from build123d import *

# Parameters (mm, degrees)
F2_R     = 2
F3_R     = 2
F4_R     = 4.6529317806
F4_R_2   = 2.3810630886
F5_DEPTH = 2.1


# Not quite as in the source:
# - a feature names something its author has since deleted; it is built from what else it names


with BuildPart() as f1:
    # F0 (on Top) → F1 (revolve)
    with BuildSketch(Plane.XY):
        with BuildLine():
            Line((12, 0), (5, 0))
            Line((5, 0), (5, 23.4674374053))
            ThreePointArc((5, 23.4674374053), (5.4354487572, 25.0240609703), (6.6153846154, 26.1287980041))
            ThreePointArc((6.6153846154, 26.1287980041), (10.5485041427, 29.8112547834), (12, 35))
            Line((12, 35), (12, 35.8777977526))
            ThreePointArc((12, 35.8777977526), (11.6461494723, 39.1166718836), (10.6012925819, 42.2027357051))
            Line((10.6012925819, 42.2027357051), (2.7202585164, 59.1502932902))
            ThreePointArc((2.7202585164, 59.1502932902), (1.6132323497, 60.414629994), (0, 60.8853056997))
            Line((0, 60.8853056997), (0, 25))
            Line((0, 25), (0, 17.2050446272))
            Line((0, 17.2050446272), (0, -4))
            Line((0, -4), (9, -4))
            Line((9, -4), (12, -4))
            Line((12, -4), (12, 0))
        make_face()
    revolve(axis=Axis((0, 21.1025223136, 0), (0, -1, 0)))

    # F2
    f2_edges = [f1.edges().sort_by_distance(p)[0] for p in [
        (-12, 0, 0),
    ]]
    fillet(f2_edges, radius=F2_R)

    # F3
    f3_edges = [f1.edges().sort_by_distance(p)[0] for p in [
        (-5, 0, 0),
    ]]
    fillet(f3_edges, radius=F3_R)

    # F4 (on Top) → F5 (cut, symmetric)
    with BuildSketch(Plane.XY):
        with Locations((0, -4.1621848941)):
            Circle(F4_R)
        with Locations((0, -4.1621848941)):
            Circle(F4_R_2, mode=Mode.SUBTRACT)
    extrude(amount=F5_DEPTH, both=True, mode=Mode.SUBTRACT)


solid = f1.part
Could you check a few things on this model? Use its own coordinates, in mm. A direction names the side the tool comes from. Round coordinates to 2 decimals unless told otherwise and drop trailing zeros. Order: outer loops, then holes, each group sorted by start corner. A loop starts at its lowest first (then second) coordinate and runs counter-clockwise, first axis right, second up.
Q1. Imagine slicing it at A-A, the plane y = 21. List the corners of the cut face in (x, z) for me.
Geometry says:
outline: circle Ø10 at (0, 0)
Q2. Please list where these lines run through material, in increasing order: probe 1 along Y at (x, z) = (-5.5, -3.75); probe 2 along Y at (x, z) = (-2, 8.75); probe 3 along X at (y, z) = (53, -2.5).
Geometry says:
probe 1: y = -4 to 0.03, 26.15 to 50.69
probe 2: y = -4 to 0, 27.83 to 45.7
probe 3: x = -4.99 to 4.99
Q3. I'm going to push flat-ended pins straight in: P1, Ø1.5, axis at y = 33.5, z = 3, coming from the -X side; P2, Ø12, axis at y = 51.5, z = 4.5, coming from the -X side; P3, Ø4, axis at y = 43.5, z = 8, coming from the -X side. Where does each tip first touch, or does it pass through?
Geometry says:
P1: stops at x = -11.7
P2: stops at x = -8.58
P3: stops at x = -8.39
Q4. Thinking about a two-plate mould opening in Y: for faces 3 (the face through (2.644, 52.678, -5.083)), 4 (the face through (-11.99, -2.99, 0.53)), 5 (the face through (0, -4, 0)), 6 (the face through (0.1, 0.49, 0.03)), which applies, released by +Y, released by -Y, zero draft, split by the parting line, or undercut?
Geometry says:
face 3: released by +Y
face 4: zero draft
face 5: released by -Y
face 6: undercut
Q5. Imagine slicing it at B-B, the plane y = 55.5. List the corners of the cut face in (x, z) for me.
Geometry says:
outline: circle Ø8.84 at (0, 0)
Q6. Which directions (+Z, -Z, +X, -X, +Y, -Y) give clear straight access to the entire face, cutting with the end or side of a thin tool? Please do faces 1 (the face through (0.05, -1.78, -0.03)), 2 (the face through (-11.99, 35.45, 0.53)).
Geometry says:
face 1: none
face 2: +Y, -Y
